```python
from build123d import *

# Parameters (mm, degrees)
SKETCH1_W           = 33.7
SKETCH1_H           = 12
BOSS_EXTRUDE1_DEPTH = 2.5
SKETCH2_W           = 33.7
SKETCH2_H           = 4.5
BOSS_EXTRUDE2_DEPTH = 17.5
SKETCH3_W           = 13
SKETCH3_H           = 23.5
CUT_EXTRUDE1_DEPTH  = 258.235074474
SKETCH4_W           = 2.85
SKETCH4_H           = 12
BOSS_EXTRUDE3_DEPTH = 23.5
FILLET1_R           = 6
SKETCH5_R           = 3
CUT_EXTRUDE2_DEPTH  = 4
SKETCH6_R           = 3.5
CUT_EXTRUDE3_DEPTH  = 4
SKETCH7_W           = 3.5
SKETCH7_H           = 12
BOSS_EXTRUDE4_DEPTH = 12
FILLET2_R           = 1
SKETCH8_R           = 0.800000001
CUT_EXTRUDE4_DEPTH  = 2


with BuildPart() as part:
    # Sketch1 → Boss-Extrude1 (new body)
    with BuildSketch(Plane(origin=(0, 0, 0), x_dir=(0, 0, -1), z_dir=(1, 0, 0))):
        with Locations((-239.496705732, 20.068965517)):
            Rectangle(SKETCH1_W, SKETCH1_H)
    extrude(amount=BOSS_EXTRUDE1_DEPTH)

    # Sketch2 → Boss-Extrude2 (add)
    with BuildSketch(Plane(origin=(2.5, 0, 0), x_dir=(0, 0, -1), z_dir=(1, 0, 0))):
        with Locations((-239.496705732, 16.318965517)):
            Rectangle(SKETCH2_W, SKETCH2_H)
    extrude(amount=BOSS_EXTRUDE2_DEPTH)

    # Sketch3 → Cut-Extrude1 (cut, through all)
    with BuildSketch(Plane(origin=(0, 18.568965517, 0), x_dir=(1, 0, 0), z_dir=(0, 1, 0))):
        with Locations((10, -239.496705732)):
            Rectangle(SKETCH3_W, SKETCH3_H)
    extrude(amount=-CUT_EXTRUDE1_DEPTH, mode=Mode.SUBTRACT)

    # Sketch4 → Boss-Extrude3 (add)
    with BuildSketch(Plane.ZY):
        with Locations((224.071705732, 20.068965517)):
            Rectangle(SKETCH4_W, SKETCH4_H)
        with Locations((254.921705732, 20.068965517)):
            Rectangle(SKETCH4_W, SKETCH4_H)
    extrude(amount=BOSS_EXTRUDE3_DEPTH)

    # Fillet1
    fillet1_edges = [part.edges().sort_by_distance(p)[0] for p in [
        (-23.5, 14.068965517, 224.071705732),
        (-23.5, 26.068965517, 224.071705732),
        (-23.5, 14.068965517, 254.921705732),
        (-23.5, 26.068965517, 254.921705732),
    ]]
    fillet(fillet1_edges, radius=FILLET1_R - 0.0001)  # a hair under: the kernel refuses the full size

    # Sketch5 → Cut-Extrude2 (cut)
    with BuildSketch(Plane.XY.offset(256.346705732)):
        with Locations((-17.5, 20.068965517)):
            Circle(SKETCH5_R)
    extrude(amount=-CUT_EXTRUDE2_DEPTH, mode=Mode.SUBTRACT)

    # Sketch6 → Cut-Extrude3 (cut)
    with BuildSketch(Plane.XY.offset(225.496705732)):
        with Locations((-17.5, 20.068965517)):
            Circle(SKETCH6_R)
    extrude(amount=-CUT_EXTRUDE3_DEPTH, mode=Mode.SUBTRACT)

    # Sketch7 → Boss-Extrude4 (add)
    with BuildSketch(Plane(origin=(0, 18.568965517, 0), x_dir=(1, 0, 0), z_dir=(0, 1, 0))):
        with Locations((1.75, -244.746705732)):
            Rectangle(SKETCH7_W, SKETCH7_H)
    extrude(amount=BOSS_EXTRUDE4_DEPTH)

    # Fillet2
    fillet2_edges = [part.edges().sort_by_distance(p)[0] for p in [
        (2.5, 22.318965517, 222.646705732),
        (11.25, 18.568965517, 256.346705732),
        (11.25, 18.568965517, 222.646705732),
        (20, 16.318965517, 256.346705732),
        (20, 14.068965517, 239.496705732),
        (20, 16.318965517, 222.646705732),
        (20, 18.568965517, 239.496705732),
        (2.5, 22.318965517, 256.346705732),
        (-21.742669976, 24.311635494, 222.646705732),
        (-21.742669976, 15.826295541, 222.646705732),
        (-21.742669976, 24.311635494, 256.346705732),
        (-21.742669976, 15.826295541, 256.346705732),
        (-7.50005, 26.068965517, 256.346705732),
        (-7.50005, 26.068965517, 222.646705732),
        (1.24995, 14.068965517, 222.646705732),
        (1.24995, 14.068965517, 256.346705732),
    ]]
    fillet(fillet2_edges, radius=FILLET2_R)

    # Sketch8 → Cut-Extrude4 (cut)
    with BuildSketch(Plane(origin=(0, 30.568965517, 0), x_dir=(1, 0, 0), z_dir=(0, 1, 0))):
        with Locations(Location((1.75, -247.746705734, 0), (0, 0, 270))):
            Circle(SKETCH8_R)
        with Locations(Location((1.75, -241.746705734, 0), (0, 0, 270))):
            Circle(SKETCH8_R)
    extrude(amount=-CUT_EXTRUDE4_DEPTH, mode=Mode.SUBTRACT)


solid = part.part
```
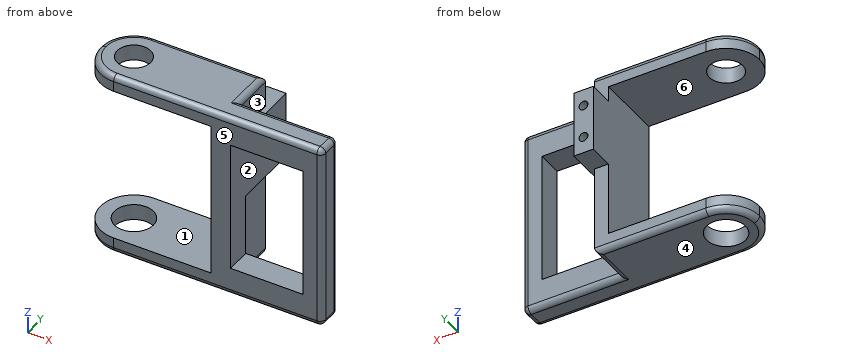
Geometry check sheet. Reference: the model listing, model coordinates, mm. Face numbers are marked on the shaded views. A direction names the side the tool comes from. Coordinates: 2 decimals unless noted, no trailing zeros. Order: outer loops, then holes, each group sorted by start corner. A loop starts at its lowest first (then second) coordinate and runs counter-clockwise, first axis right, second up. Notation, with made-up numbers: (51.25, -25) - (105.25, -25) arc R14 cw to (105.25, -7) - close; hole circle Ø3 at (72.25, -30.5). An arc over 180 degrees is marked (long way). Answer as a JSON object with one key per item and string values. Group by question number.
Item 1: Sectioned sample at C-C, the plane y = 28. Record the cut outline in (x, z), and give its area (3 significant figures).
Item 2: Sectioned sample at B-B, the plane z = 228.5. Record the cut outline in (x, y), and give its area (3 significant figures).
Item 3: Scan lines: probe 1 along Z at (x, y) = (4, 16.75); probe 2 along Z at (x, y) = (-3.5, 15); probe 3 along Y at (x, z) = (-17.5, 224.4). Record each from-to range of solid material in increasing order.
Item 4: Draft check along Z on the marked faces 4, 5 and 6. Enter one of: +Z half, -Z half, draft (parallel to the pull), parting line (faces both ways), or undercut.
Item 5: Sectioned sample at A-A, the plane x = -12. Record the cut outline in (y, z), and give its area (3 significant figures).
Item 6: Tool access check on the marked faces 1, 2 and 3. Record the directions out of +Z, -Z, +X, -X, +Y, -Y that give a thin tool (end or side, any length) a straight path to the whole face; none if there is none.
Item 7: Sectioned sample at D-D, the plane x = -19.5. Give the number of separate pieces and of enclosed holes in the cut face, and give its area (3 significant figures).
Item 8: Depth check by flat-ended pin: pin 1 Ø0.5 at (x, z) = (2, 241.5) entering from +Y; pin 2 Ø3.5 at (y, z) = (22, 254) entering from +X; pin 3 Ø3 at (y, z) = (25.5, 248.5) entering from +X. Enter the tip coordinate at first touch or a pass-through.
Resolved:
{
 "1": {"outline": "(0, 238.75) - (3.5, 238.75) - (3.5, 250.75) - (0, 250.75) - close", "area": "42.0 mm^2"},
 "2": {"outline": "(0, 14.07) - (3.5, 14.07) - (3.5, 18.57) - (2.5, 18.57) - (2.5, 26.07) - (0, 26.07) - close; (16.5, 14.07) - (19, 14.07) arc R1 ccw to (20, 15.07) - (20, 17.57) arc R1 ccw to (19, 18.57) - (16.5, 18.57) - close", "area": "49.8 mm^2"},
 "3": {"probe 1": "222.65 to 227.75, 251.25 to 256.35", "probe 2": "222.65 to 225.5, 253.5 to 256.34", "probe 3": "14.07 to 16.57, 23.57 to 26.07"},
 "4": {"face 4": "-Z half", "face 5": "draft", "face 6": "undercut"},
 "5": {"outline": "(14.07, 223.65) arc R1 ccw to (15.07, 222.65) - (25.07, 222.65) arc R1 ccw to (26.07, 223.65) - (26.07, 225.5) - (14.07, 225.5) - close; (14.07, 253.5) - (26.07, 253.5) - (26.07, 255.35) arc R1 ccw to (25.07, 256.35) - (15.07, 256.35) arc R1 ccw to (14.07, 255.35) - close", "area": "67.5 mm^2"},
 "6": {"face 1": "-X, +Y, -Y", "face 2": "+Y, -Y", "face 3": "+Z, +X, +Y"},
 "7": {"separate pieces": "4", "enclosed holes": "0", "area": "34.5 mm^2"},
 "8": {"pin 1": "y = 28.57", "pin 2": "x = 2.5", "pin 3": "x = 3.5"}
}
